```python
from build123d import *

# Parameters (mm, degrees)
ESQUISSE1_R        = 50
ESQUISSE1_R_2      = 3
ESQUISSE1_W        = 73.2
ESQUISSE1_H        = 62.5
BOSS_EXTRU_1_DEPTH = 5


with BuildPart() as part:
    # Esquisse1 → Boss.-Extru.1 (new body)
    with BuildSketch(Plane.XY):
        Circle(ESQUISSE1_R)
        with Locations((43, 0)):
            Circle(ESQUISSE1_R_2, mode=Mode.SUBTRACT)
        with Locations((0, 43)):
            Circle(ESQUISSE1_R_2, mode=Mode.SUBTRACT)
        with Locations((-43, 0)):
            Circle(ESQUISSE1_R_2, mode=Mode.SUBTRACT)
        with Locations((0, -43)):
            Circle(ESQUISSE1_R_2, mode=Mode.SUBTRACT)
        Rectangle(ESQUISSE1_W, ESQUISSE1_H, mode=Mode.SUBTRACT)
    extrude(amount=BOSS_EXTRU_1_DEPTH)


solid = part.part
```
The model under review builds one solid part; all positions refer to its coordinate system, in mm. A direction names the side the tool comes from. Round coordinates to 2 decimals unless told otherwise and drop trailing zeros. Loops run counter-clockwise (first coordinate to the right, second up) from the corner with the lowest first, then second, coordinate; pieces in that order, holes last. Notation, with made-up numbers: (78, 78) - (90, 78) arc R31 ccw to (90, 116) - close; hole circle Ø5 at (8.25, 64). An arc over 180 degrees is marked (long way). Use a Markdown table: item, result. Add a question column.
Q1. Add section D-D (y = -19). State the section outline as (x, z) points, plus the area to 3 significant figures.
Q2. Add section B-B (y = 0). State the section outline as (x, z) points.
Q3. For probe 1 along Y at (x, z) = (0, 3); probe 2 along X at (y, z) = (28.5, 4.3); probe 3 along Y at (x, z) = (29.5, 2.2), list the stretches that pass through material, from the lowest coordinate up.
Q4. Insertion check: pin 1 Ø2 at (y, z) = (-15, 4) entering from +X; pin 2 Ø1.5 at (x, z) = (1.5, 3.5) entering from +Y; pin 3 Ø5 at (x, y) = (0, -43) entering from -Z; pin 4 Ø1 at (x, z) = (24, 0.5) entering from -Y. Each pin has a flat end and moves straight along its axis. Give the tip position at first contact, or say it passes through.
Q5. Add section A-A (x = 0). State the section outline as (y, z) points, plus the area to 4 significant figures.
Q6. The part is to be moulded in two halves that separate along X. For faces 1 (the face through (0, 34, 0)), 2 (the face through (36.6, 0, 2)), 3 (the face through (47.69, 15.02, 2.46)), say which applies: pulls with the +X half, pulls with the -X half, needs draft (parallel to the pull), parting line crosses it, or undercut.
Q7. Add section C-C (z = 3.7). State the section outline as (x, y) points.
Q8. Machinability: for faces 4 (the face through (0, 34, 5)), 5 (the face through (-1, 31.25, 2)), which of the approach directions +Z, -Z, +X, -X, +Y, -Y give a long, thin tool a straight path to every point of the face, cutting with its end or side? Answer none if there is none.
Worked answers:
| question | item | result |
|---|---|---|
| 1 | outline | (-46.25, 0) - (-36.6, 0) - (-36.6, 5) - (-46.25, 5) - close; (36.6, 0) - (46.25, 0) - (46.25, 5) - (36.6, 5) - close |
| 1 | area | 96.5 mm² |
| 2 | outline | (-50, 0) - (-46, 0) - (-46, 5) - (-50, 5) - close; (-40, 0) - (-36.6, 0) - (-36.6, 5) - (-40, 5) - close; (36.6, 0) - (40, 0) - (40, 5) - (36.6, 5) - close; (46, 0) - (50, 0) - (50, 5) - (46, 5) - close |
| 3 | probe 1 | -50 to -46, -40 to -31.25, 31.25 to 40, 46 to 50 |
| 3 | probe 2 | -41.08 to -36.6, 36.6 to 41.08 |
| 3 | probe 3 | -40.37 to -31.25, 31.25 to 40.37 |
| 4 | pin 1 | x = 48 |
| 4 | pin 2 | y = 49.99 |
| 4 | pin 3 | through |
| 4 | pin 4 | y = -44.13 |
| 5 | outline | (-50, 0) - (-46, 0) - (-46, 5) - (-50, 5) - close; (-40, 0) - (-31.25, 0) - (-31.25, 5) - (-40, 5) - close; (31.25, 0) - (40, 0) - (40, 5) - (31.25, 5) - close; (46, 0) - (50, 0) - (50, 5) - (46, 5) - close |
| 5 | area | 127.5 mm² |
| 6 | face 1 | needs draft |
| 6 | face 2 | undercut |
| 6 | face 3 | parting line crosses it |
| 7 | outline | circle Ø100 at (0, 0); hole circle Ø6 at (-43, 0); hole (-36.6, -31.25) - (36.6, -31.25) - (36.6, 31.25) - (-36.6, 31.25) - close; hole circle Ø6 at (0, -43); hole circle Ø6 at (0, 43); hole circle Ø6 at (43, 0) |
| 8 | face 4 | +Z, +X, -X, +Y, -Y |
| 8 | face 5 | +Z, -Z |
